Build history of the part. All positions in model axes, mm. A direction names the side the tool comes from. Coordinates: 2 decimals unless noted, no trailing zeros. Order: outer loops, then holes, each group sorted by start corner. A loop starts at its lowest first (then second) coordinate and runs counter-clockwise, first axis right, second up. Notation, with made-up numbers: M 78.25,-19.75 L 86.25,-19.75 A29 ccw 86.25,10.25 Z; hole C 6,39.5 d6. An arc over 180 degrees is marked long. Write item = value, one per line. Start each with the question number.
Q1. Band-saw the part on C-C on x = 10.5. Write the cut outline in (y, z) (3 decimals), plus the area to 3 significant figures.
Q2. Band-saw the part on B-B on z = 15.25. Write the cut outline in (x, y) (3 decimals), plus the area to 3 significant figures.
Q3. Drill centre lines: probe 1 along X at (y, z) = (3.5, 16.25); probe 2 along Z at (x, y) = (19.25, 7.5). Where is each one in solid material? Low to high.
Q4. 3-axis set-ups, long thin cutter, end or side, ignore diameter. For faces 1 (the face through (10, 11, 0)), 2 (the face through (12, 11, 3)): which of +Z, -Z, +X, -X, +Y, -Y reach the whole face in a straight line?
Q5. Band-saw the part on A-A on y = 16.5. Write the cut outline in (x, z).
Q6. Pin check, flat tips, straight feed: P1, Ø2, axis at x = 17, z = 5.5, coming from the -Y side; P2, Ø1.5, axis at y = 6.5, z = 21, coming from the +X side; P3, Ø3, axis at y = 9.5, z = 4, coming from the +X side; P4, Ø3.5, axis at x = 10.5, y = 12.5, coming from the +Z side. Stop position of each tip, or through.
Solid Edge part; units mm, degrees
sketch "Sketch1" plane through (0, 0, 0) normal (0, -1, 0) x (1, 0, 0)
  line L0 (20, 0) -> (20, 1)
  arc A0 (18, 3) -> (20, 1) centre (18, 1) cw
  line L1 (18, 3) -> (6.5, 3)
  arc A1 (3, 6.5) -> (6.5, 3) centre (6.5, 6.5) ccw
  line L2 (3, 6.5) -> (3, 28)
  arc A2 (1, 30) -> (3, 28) centre (1, 28) cw
  line L3 (1, 30) -> (0, 30)
  line L4 (0, 30) -> (0, 0)
  line L5 (0, 0) -> (20, 0)
extrude "Protrusion1" add sketch "Sketch1" against normal blind 22.225
Recorded:
q1.outline = M 0,0 L 22.225,0 L 22.225,3 L 0,3 Z
q1.area = 66.7 mm2
q2.outline = M 0,0 L 3,0 L 3,22.225 L 0,22.225 Z
q2.area = 66.7 mm2
q3.probe_1 = 0 to 3
q3.probe_2 = 0 to 2.56
q4.face_1 = -Z, +X, -X, +Y, -Y
q4.face_2 = +Z, +X, +Y, -Y
q5.outline = M 0,0 L 20,0 L 20,1 A2 ccw 18,3 L 6.5,3 A3.5 cw 3,6.5 L 3,28 A2 ccw 1,30 L 0,30 Z
q6.P1 = through
q6.P2 = 3
q6.P3 = 19.32
q6.P4 = 3
